Verification items for the finished model (mm, model axes). A direction names the side the tool comes from. Give positions to 0.01 mm unless a question says otherwise; leave off trailing zeros. Loops run counter-clockwise (first coordinate to the right, second up) from the corner with the lowest first, then second, coordinate; pieces in that order, holes last. Notation, with made-up numbers: (6.5, 23.5) - (30.5, 23.5) arc R18 cw to (30.5, 35.5) - close; hole circle Ø2 at (27.5, 60). An arc over 180 degrees is marked (long way). One line per question, with ' | ' between items. Start each with the question number.
1. Depth check by flat-ended pin: pin 1 Ø6 at (y, z) = (-27.5, 67.5) entering from -X; pin 2 Ø2 at (x, z) = (-98.5, 99) entering from +Y; pin 3 Ø3 at (x, z) = (-169.5, -50.5) entering from +Y; pin 4 Ø15 at (y, z) = (0, 65) entering from +X. Enter the tip coordinate at first touch or a pass-through.
2. Mould release check, pull along Z, two halves, no side actions. Record for faces 5 (the face through (250, -1, 2)), 6 (the face through (207, -10.1, -55)): +Z half, -Z half, draft (parallel to the pull), parting line (faces both ways), or undercut.
3. Section check B-B, the plane y = -25. State how many separate pieces and enclosed holes the cut face has, then the cut area to 3 significant figures.
4. Tool access check on faces 1 (the face through (247.54, 1.4, 96.72)), 2 (the face through (-163, 85, -2)), 3 (the face through (-207, -46, 18.85)), 4 (the face through (-245, -14, 65)). Record the directions out of +Z, -Z, +X, -X, +Y, -Y that give a thin tool (end or side, any length) a straight path to the whole face; none if there is none.
5. Section check A-A, the plane x = -72. Enter the section's corners in (y, z), then the cut area to 3 significant figures.
6. Thickness scan on line 1 along X through (y, z) = (80.25, 100); line 2 along X through (y, z) = (-41, 33); line 3 along X through (y, z) = (-86, 100). Record the ranges inside material, lowest first. Write a range as from..to.
from build123d import *

# Parameters (mm, degrees)
SKETCH1_W                      = 250
SKETCH1_H                      = 200
BOSS_EXTRUDE1_DEPTH            = 250
SKETCH7_W                      = 470
SKETCH7_H                      = 230
CUT_EXTRUDE4_DEPTH             = 80
SKETCH5_R                      = 31.75
F_63_5MM_DIA_SERVO_DEPTH       = 5
MIRROR13_COPY_1_SKETCH_R       = 31.75
MIRROR13_COPY_1_DEPTH          = 5
SKETCH10_W                     = 350
SKETCH10_H                     = 220
CUT_EXTRUDE5_DEPTH             = 20
SKETCH15_W                     = 500
SKETCH15_H                     = 250
BOSS_EXTRUDE2_DEPTH            = 10
SKETCH18_W                     = 300
SKETCH18_H                     = 220
CUT_EXTRUDE11_DEPTH            = 10
SKETCH19_R                     = 3.5
CUT_EXTRUDE12_DEPTH            = 10
MIRROR15_COPY_1_SKETCH_R       = 3.5
MIRROR15_COPY_1_DEPTH          = 10
SKETCH20_R                     = 3.5
CUT_EXTRUDE13_DEPTH            = 10
MIRROR17_COPY_1_SKETCH_R       = 3.5
MIRROR17_COPY_1_DEPTH          = 10
SKETCH22_R                     = 12.55
CUT_EXTRUDE14_DEPTH            = 10
MIRROR19_COPY_1_SKETCH_R       = 12.55
MIRROR19_COPY_1_DEPTH          = 10
SKETCH23_W                     = 22.35
SKETCH23_H                     = 72
BOSS_EXTRUDE3_DEPTH            = 69.9
MIRROR21_COPY_1_SKETCH_W       = 22.35
MIRROR21_COPY_1_SKETCH_H       = 72
MIRROR21_COPY_1_DEPTH          = 69.9
F_1_0MM_DOWEL_HOLE1_AT_2_COUNT = 2
F_1_0MM_DOWEL_HOLE1_AT_2_PITCH = 8
F_1_0MM_DOWEL_HOLE1_AT_3_COUNT = 2
F_1_0MM_DOWEL_HOLE1_AT_3_PITCH = 65.49045732
F_1_0MM_DOWEL_HOLE1_AT_4_COUNT = 2
F_1_0MM_DOWEL_HOLE1_AT_4_PITCH = 65


with BuildPart() as part:
    # Sketch1 → Boss-Extrude1 (new, symmetric)
    with BuildSketch(Plane(origin=(0, 0, 0), x_dir=(0, 0, -1), z_dir=(1, 0, 0))):
        Rectangle(SKETCH1_W, SKETCH1_H)
    extrude(amount=BOSS_EXTRUDE1_DEPTH, both=True)

    # Sketch7 → Cut-Extrude4 (cut, symmetric)
    with BuildSketch(Plane(origin=(0, 0, 0), x_dir=(1, 0, 0), z_dir=(0, 1, 0))):
        Rectangle(SKETCH7_W, SKETCH7_H)
    extrude(amount=CUT_EXTRUDE4_DEPTH, both=True, mode=Mode.SUBTRACT)

    # Sketch5 → 63.5mm_dia_servo (cut)
    with BuildSketch(Plane(origin=(250, 0, 0), x_dir=(0, 0, -1), z_dir=(1, 0, 0))):
        with Locations((-65, 0)):
            Circle(SKETCH5_R)
    f_63_5mm_dia_servo = extrude(amount=-F_63_5MM_DIA_SERVO_DEPTH, mode=Mode.SUBTRACT)

    # Mirror12: 63.5mm_dia_servo across plane
    add(f_63_5mm_dia_servo.mirror(Plane.XY), mode=Mode.SUBTRACT)

    # Mirror13: 63.5mm_dia_servo across plane
    add(f_63_5mm_dia_servo.mirror(Plane(origin=(0, 0, 0), x_dir=(0, 0, 1), z_dir=(1, 0, 0))), mode=Mode.SUBTRACT)

    # Mirror13 copy 1 sketch → Mirror13 copy 1 (cut)
    with BuildSketch(Plane.ZY.offset(250)):
        with Locations((-65, 0)):
            Circle(MIRROR13_COPY_1_SKETCH_R)
    extrude(amount=-MIRROR13_COPY_1_DEPTH, mode=Mode.SUBTRACT)

    # Sketch10 → Cut-Extrude5 (cut)
    with BuildSketch(Plane(origin=(0, 100, 0), x_dir=(1, 0, 0), z_dir=(0, 1, 0))):
        Rectangle(SKETCH10_W, SKETCH10_H)
    extrude(amount=-CUT_EXTRUDE5_DEPTH, mode=Mode.SUBTRACT)

    # Sketch15 → Boss-Extrude2 (add)
    with BuildSketch(Plane(origin=(0, 75, 0), x_dir=(1, 0, 0), z_dir=(0, 1, 0))):
        Rectangle(SKETCH15_W, SKETCH15_H)
    extrude(amount=BOSS_EXTRUDE2_DEPTH)

    # Sketch18 → Cut-Extrude11 (cut)
    with BuildSketch(Plane(origin=(0, 85, 0), x_dir=(1, 0, 0), z_dir=(0, 1, 0))):
        Rectangle(SKETCH18_W, SKETCH18_H)
    extrude(amount=-CUT_EXTRUDE11_DEPTH, mode=Mode.SUBTRACT)

    # Sketch19 → Cut-Extrude12 (cut)
    with BuildSketch(Plane(origin=(0, 85, 0), x_dir=(1, 0, 0), z_dir=(0, 1, 0))):
        with Locations(Location((-162.5, 100, 0), (0, 0, 270))):
            Circle(SKETCH19_R)
    cut_extrude12 = extrude(amount=-CUT_EXTRUDE12_DEPTH, mode=Mode.SUBTRACT)

    # Mirror14: Cut-Extrude12 across plane
    add(cut_extrude12.mirror(Plane.XY), mode=Mode.SUBTRACT)

    # Mirror15: Cut-Extrude12 across plane
    add(cut_extrude12.mirror(Plane(origin=(0, 0, 0), x_dir=(0, 0, 1), z_dir=(1, 0, 0))), mode=Mode.SUBTRACT)

    # Mirror15 copy 1 sketch → Mirror15 copy 1 (cut)
    with BuildSketch(Plane(origin=(0, 85, 0), x_dir=(-1, 0, 0), z_dir=(0, 1, 0))):
        with Locations(Location((-162.5, 100, 0), (0, 0, 270))):
            Circle(MIRROR15_COPY_1_SKETCH_R)
    extrude(amount=-MIRROR15_COPY_1_DEPTH, mode=Mode.SUBTRACT)

    # Sketch20 → Cut-Extrude13 (cut)
    with BuildSketch(Plane(origin=(0, -80, 0), x_dir=(1, 0, 0), z_dir=(0, 1, 0))):
        with Locations(Location((-100, 100, 0), (0, 0, 270))):
            Circle(SKETCH20_R)
    cut_extrude13 = extrude(amount=-CUT_EXTRUDE13_DEPTH, mode=Mode.SUBTRACT)

    # Mirror16: Cut-Extrude13 across plane
    add(cut_extrude13.mirror(Plane.XY), mode=Mode.SUBTRACT)

    # Mirror17: Cut-Extrude13 across plane
    add(cut_extrude13.mirror(Plane(origin=(0, 0, 0), x_dir=(0, 0, 1), z_dir=(1, 0, 0))), mode=Mode.SUBTRACT)

    # Mirror17 copy 1 sketch → Mirror17 copy 1 (cut)
    with BuildSketch(Plane(origin=(0, -80, 0), x_dir=(-1, 0, 0), z_dir=(0, 1, 0))):
        with Locations(Location((-100, 100, 0), (0, 0, 270))):
            Circle(MIRROR17_COPY_1_SKETCH_R)
    extrude(amount=-MIRROR17_COPY_1_DEPTH, mode=Mode.SUBTRACT)

    # Sketch22 → Cut-Extrude14 (cut)
    with BuildSketch(Plane(origin=(245, 0, 0), x_dir=(0, 0, -1), z_dir=(1, 0, 0))):
        with Locations((-65, 0)):
            Circle(SKETCH22_R)
    cut_extrude14 = extrude(amount=-CUT_EXTRUDE14_DEPTH, mode=Mode.SUBTRACT)

    # Mirror18: Cut-Extrude14 across plane
    add(cut_extrude14.mirror(Plane(origin=(0, 0, 0), x_dir=(0, 0, 1), z_dir=(1, 0, 0))), mode=Mode.SUBTRACT)

    # Mirror19: Cut-Extrude14 across plane
    add(cut_extrude14.mirror(Plane.XY), mode=Mode.SUBTRACT)

    # Mirror19 copy 1 sketch → Mirror19 copy 1 (cut)
    with BuildSketch(Plane.ZY.offset(245)):
        with Locations((-65, 0)):
            Circle(MIRROR19_COPY_1_SKETCH_R)
    extrude(amount=-MIRROR19_COPY_1_DEPTH, mode=Mode.SUBTRACT)

    # Sketch23 → Boss-Extrude3 (add)
    with BuildSketch(Plane(origin=(0, -80, 0), x_dir=(1, 0, 0), z_dir=(0, 1, 0))):
        with Locations((207.175, 54.85)):
            Rectangle(SKETCH23_W, SKETCH23_H)
    boss_extrude3 = extrude(amount=BOSS_EXTRUDE3_DEPTH)

    # Mirror20: Boss-Extrude3 across plane
    add(boss_extrude3.mirror(Plane(origin=(0, 0, 0), x_dir=(0, 0, 1), z_dir=(1, 0, 0))))

    # Mirror21: Boss-Extrude3 across plane
    add(boss_extrude3.mirror(Plane.XY))

    # Mirror21 copy 1 sketch → Mirror21 copy 1 (add)
    with BuildSketch(Plane(origin=(0, -80, 0), x_dir=(-1, 0, 0), z_dir=(0, 1, 0))):
        with Locations((207.175, 54.85)):
            Rectangle(MIRROR21_COPY_1_SKETCH_W, MIRROR21_COPY_1_SKETCH_H)
    extrude(amount=MIRROR21_COPY_1_DEPTH)

    # Sketch29 → Ø1.0mm Dowel Hole1 (revolve, cut)
    with BuildSketch(Plane(origin=(-214.35, -10.1, -87.35), x_dir=(0, 0, 1), z_dir=(1, 0, 0))):
        Polygon((0, 0), (0, 9.201721238), (2, 8), (2, 0), align=None)
    f_1_0mm_dowel_hole1 = revolve(axis=Axis((-214.35, -3.75, -87.35), (0, -1, 0)), mode=Mode.SUBTRACT)

    # Ø1.0mm Dowel Hole1 at 2: Ø1.0mm Dowel Hole1 ×2
    with Locations(*[(i * F_1_0MM_DOWEL_HOLE1_AT_2_PITCH, 0, 0) for i in range(1, F_1_0MM_DOWEL_HOLE1_AT_2_COUNT)]):
        add(f_1_0mm_dowel_hole1, mode=Mode.SUBTRACT)

    # Ø1.0mm Dowel Hole1 at 3: Ø1.0mm Dowel Hole1 ×2
    with Locations(*[Vector(0.12215520134321664, 0, 0.9925110109136313) * (i * F_1_0MM_DOWEL_HOLE1_AT_3_PITCH) for i in range(1, F_1_0MM_DOWEL_HOLE1_AT_3_COUNT)]):
        add(f_1_0mm_dowel_hole1, mode=Mode.SUBTRACT)

    # Ø1.0mm Dowel Hole1 at 4: Ø1.0mm Dowel Hole1 ×2
    with Locations(*[(0, 0, i * F_1_0MM_DOWEL_HOLE1_AT_4_PITCH) for i in range(1, F_1_0MM_DOWEL_HOLE1_AT_4_COUNT)]):
        add(f_1_0mm_dowel_hole1, mode=Mode.SUBTRACT)

    # Mirror22: Ø1.0mm Dowel Hole1 across plane
    add(f_1_0mm_dowel_hole1.mirror(Plane.XY), mode=Mode.SUBTRACT)

    # Mirror22 copy 1 sketch → Mirror22 copy 1 (revolve, cut)
    with BuildSketch(Plane(origin=(-206.35, -10.1, 87.35), x_dir=(0, 0, -1), z_dir=(1, 0, 0))):
        Polygon((0, 0), (0, -9.201721238), (2, -8), (2, 0), align=None)
    revolve(axis=Axis((-206.35, -3.75, 87.35), (0, 1, 0)), mode=Mode.SUBTRACT)

    # Mirror22 copy 2 sketch → Mirror22 copy 2 (revolve, cut)
    with BuildSketch(Plane(origin=(-206.35, -10.1, 22.35), x_dir=(0, 0, -1), z_dir=(1, 0, 0))):
        Polygon((0, 0), (0, -9.201721238), (2, -8), (2, 0), align=None)
    revolve(axis=Axis((-206.35, -3.75, 22.35), (0, 1, 0)), mode=Mode.SUBTRACT)

    # Mirror22 copy 3 sketch → Mirror22 copy 3 (revolve, cut)
    with BuildSketch(Plane(origin=(-214.35, -10.1, 22.35), x_dir=(0, 0, -1), z_dir=(1, 0, 0))):
        Polygon((0, 0), (0, -9.201721238), (2, -8), (2, 0), align=None)
    revolve(axis=Axis((-214.35, -3.75, 22.35), (0, 1, 0)), mode=Mode.SUBTRACT)

    # Mirror23: Ø1.0mm Dowel Hole1 across plane
    add(f_1_0mm_dowel_hole1.mirror(Plane(origin=(0, 0, 0), x_dir=(0, 0, 1), z_dir=(1, 0, 0))), mode=Mode.SUBTRACT)

    # Mirror23 copy 1 sketch → Mirror23 copy 1 (revolve, cut)
    with BuildSketch(Plane(origin=(206.35, -10.1, -87.35), x_dir=(0, 0, 1), z_dir=(-1, 0, 0))):
        Polygon((0, 0), (0, -9.201721238), (2, -8), (2, 0), align=None)
    revolve(axis=Axis((206.35, -3.75, -87.35), (0, 1, 0)), mode=Mode.SUBTRACT)

    # Mirror23 copy 2 sketch → Mirror23 copy 2 (revolve, cut)
    with BuildSketch(Plane(origin=(206.35, -10.1, -22.35), x_dir=(0, 0, 1), z_dir=(-1, 0, 0))):
        Polygon((0, 0), (0, -9.201721238), (2, -8), (2, 0), align=None)
    revolve(axis=Axis((206.35, -3.75, -22.35), (0, 1, 0)), mode=Mode.SUBTRACT)

    # Mirror23 copy 3 sketch → Mirror23 copy 3 (revolve, cut)
    with BuildSketch(Plane(origin=(214.35, -10.1, -22.35), x_dir=(0, 0, 1), z_dir=(-1, 0, 0))):
        Polygon((0, 0), (0, -9.201721238), (2, -8), (2, 0), align=None)
    revolve(axis=Axis((214.35, -3.75, -22.35), (0, 1, 0)), mode=Mode.SUBTRACT)

    # Mirror23 copy 4 sketch → Mirror23 copy 4 (revolve, cut)
    with BuildSketch(Plane(origin=(214.35, -10.1, 87.35), x_dir=(0, 0, -1), z_dir=(-1, 0, 0))):
        Polygon((0, 0), (0, 9.201721238), (2, 8), (2, 0), align=None)
    revolve(axis=Axis((214.35, -3.75, 87.35), (0, -1, 0)), mode=Mode.SUBTRACT)

    # Mirror23 copy 5 sketch → Mirror23 copy 5 (revolve, cut)
    with BuildSketch(Plane(origin=(206.35, -10.1, 87.35), x_dir=(0, 0, -1), z_dir=(-1, 0, 0))):
        Polygon((0, 0), (0, 9.201721238), (2, 8), (2, 0), align=None)
    revolve(axis=Axis((206.35, -3.75, 87.35), (0, -1, 0)), mode=Mode.SUBTRACT)

    # Mirror23 copy 6 sketch → Mirror23 copy 6 (revolve, cut)
    with BuildSketch(Plane(origin=(206.35, -10.1, 22.35), x_dir=(0, 0, -1), z_dir=(-1, 0, 0))):
        Polygon((0, 0), (0, 9.201721238), (2, 8), (2, 0), align=None)
    revolve(axis=Axis((206.35, -3.75, 22.35), (0, -1, 0)), mode=Mode.SUBTRACT)

    # Mirror23 copy 7 sketch → Mirror23 copy 7 (revolve, cut)
    with BuildSketch(Plane(origin=(214.35, -10.1, 22.35), x_dir=(0, 0, -1), z_dir=(-1, 0, 0))):
        Polygon((0, 0), (0, 9.201721238), (2, 8), (2, 0), align=None)
    revolve(axis=Axis((214.35, -3.75, 22.35), (0, -1, 0)), mode=Mode.SUBTRACT)


solid = part.part
Results list:
1) pin 1: x = -245 | pin 2: y = -90 | pin 3: y = 85 | pin 4: through
2) face 5: draft | face 6: undercut
3) separate pieces: 5 | enclosed holes: 1 | area: 22,600 mm²
4) face 1: +X | face 2: +Y | face 3: none | face 4: -X
5) outline: (-100, -125) - (100, -125) - (100, -110) - (75, -110) - (75, -115) - (-80, -115) - (-80, 115) - (75, 115) - (75, 110) - (100, 110) - (100, 125) - (-100, 125) - close | area: 8,850 mm²
6) line 1: -250..-166, -159..-150, 150..159, 166..250 | line 2: -250..-235, -218.35..-196, 196..218.35, 235..250 | line 3: -250..-103.5, -96.5..96.5, 103.5..250
